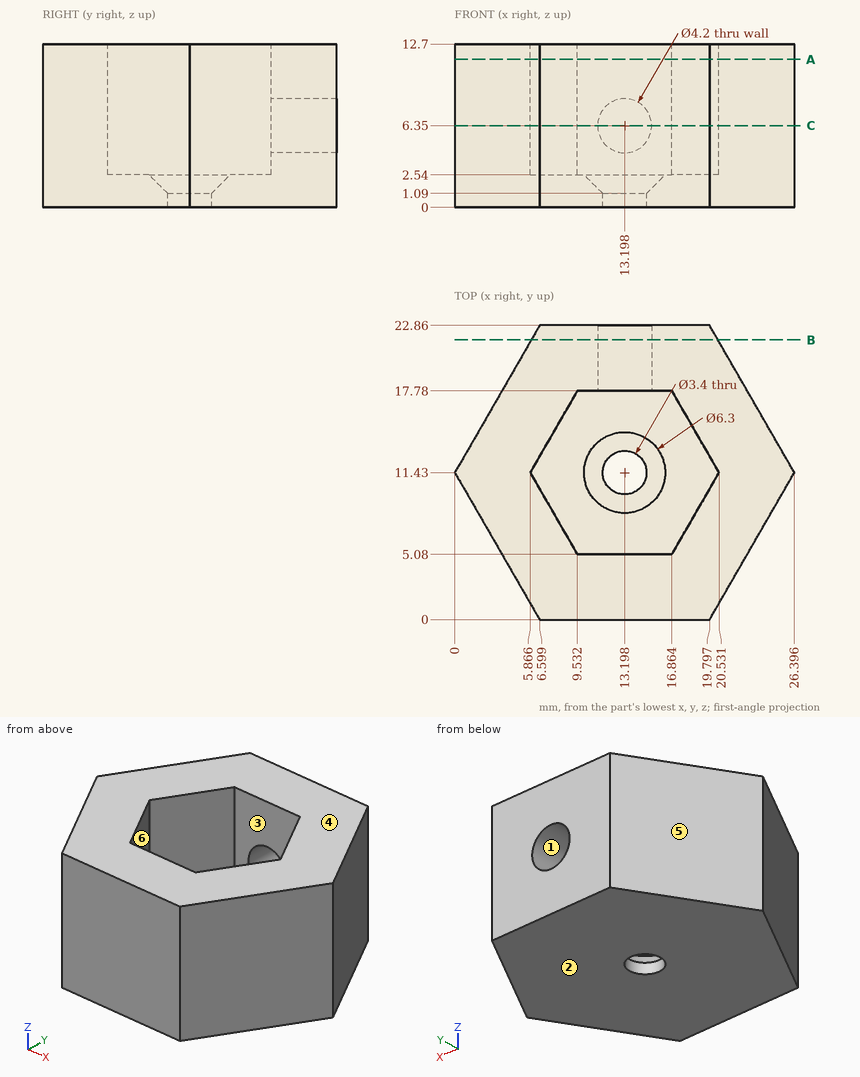
Drawing for the job (mm, zero at the part's lowest x, y, z). A direction names the side the tool comes from. Give positions to 0.01 mm unless a question says otherwise; leave off trailing zeros. Write each loop counter-clockwise with the first axis right and the second up, starting at its lowest first coordinate (ties: lowest second). Pieces come first, ordered by that corner, then holes. Notation, with made-up numbers: M 52,-2.75 L 77,-2.75 A19 ccw 77,32.25 Z; hole C 86,49 d7. An arc over 180 degrees is marked long. Use CSV: the item, a comma, the result in double quotes.
Item 1: Slice it at A-A on z = 11.5. Write the cut outline in (x, y) (1 decimal).
Taken from the geometry:
outline,"M 0,11.4 L 6.6,0 L 19.8,0 L 26.4,11.4 L 19.8,22.9 L 6.6,22.9 Z; hole M 5.9,11.4 L 9.5,5.1 L 16.9,5.1 L 20.5,11.4 L 16.9,17.8 L 9.5,17.8 Z"
Item 2: Which spindle directions (+Z, -Z, +X, -X, +Y, -Y) get a long thin tool onto all of the face, cutting with end or side? Do the marked faces 5 and 6. Say none if no direction does.
Taken from the geometry:
face 5,"+Z, -Z, -X, +Y"
face 6,"+Z"
Item 3: Drill centre lines: probe 1 along Y at (x, z) = (12, 8.5); probe 2 along Y at (x, z) = (6, 8) (1 decimal); probe 3 along X at (y, z) = (14.75, 7.5) (1 decimal). Where is each one in solid material? Low to high.
Taken from the geometry:
probe 1,"y = 0 to 5.08, 17.78 to 22.86"
probe 2,"y = 1 to 11.2, 11.7 to 21.8"
probe 3,"x = 1.9 to 7.8, 18.6 to 24.5"
Item 4: Slice it at B-B on y = 21.75. Write the cut outline in (x, z).
Taken from the geometry:
outline,"M 5.96,0 L 20.44,0 L 20.44,12.7 L 5.96,12.7 Z; hole C 13.2,6.35 d4.2"
Item 5: Pull direction Z, two halves, no side cores. Call the marked faces 1, 2, 3 and 4: +Z half, -Z half, draft (parallel to the pull), parting line (faces both ways), or undercut.
Taken from the geometry:
face 1,"undercut"
face 2,"-Z half"
face 3,"draft"
face 4,"+Z half"
Item 6: Slice it at C-C on z = 6.35. Write the cut outline in (x, y) (1 decimal).
Taken from the geometry:
outline,"M 0,11.4 L 6.6,0 L 19.8,0 L 26.4,11.4 L 19.8,22.9 L 15.3,22.9 L 15.3,17.8 L 16.9,17.8 L 20.5,11.4 L 16.9,5.1 L 9.5,5.1 L 5.9,11.4 L 9.5,17.8 L 11.1,17.8 L 11.1,22.9 L 6.6,22.9 Z"
Item 7: Pin check, flat tips, straight feed: P1, Ø10, axis at x = 16.5, y = 10, coming from the +Z side; P2, Ø4, axis at y = 9, z = 3.5, coming from the +X side; P3, Ø5, axis at x = 22.5, z = 6, coming from the +Y side; P4, Ø4.5, axis at x = 13.2, y = 11.43, coming from the +Z side. Stop position of each tip, or through.
Taken from the geometry:
P1,"stops at z = 12.7"
P2,"stops at x = 26.15"
P3,"stops at y = 22.51"
P4,"stops at z = 1.64"
